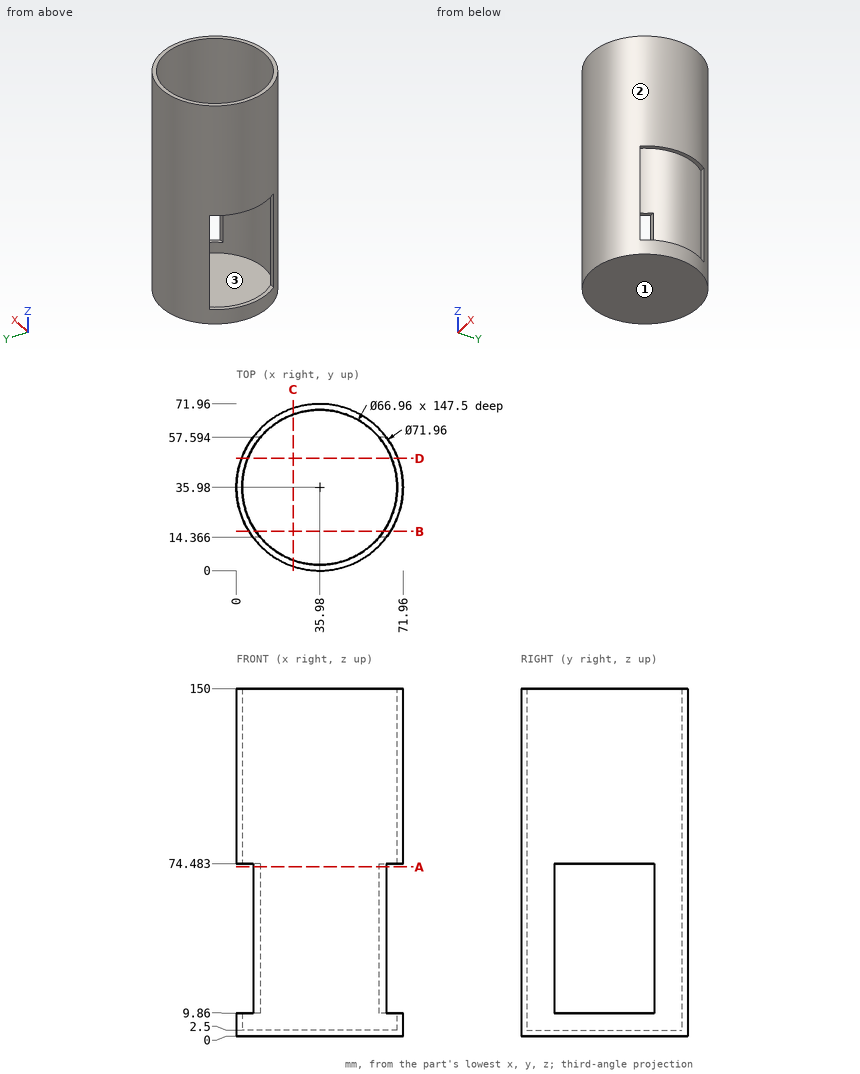
Could you check a few things on this drawing? It's one solid part, dimensions in mm from its lowest x, y, z. Give positions to 0.01 mm unless a question says otherwise; leave off trailing zeros. Order: outer loops, then holes, each group sorted by start corner. A loop starts at its lowest first (then second) coordinate and runs counter-clockwise, first axis right, second up. Notation, with made-up numbers: (-27, 20.5) - (20, 20.5) arc R6 ccw to (20, 29.5) - close; hole circle Ø1 at (64.5, 62). An arc over 180 degrees is marked (long way). Return JSON: item names as keys, results as strings. Group by question number.
Q1. Thinking about a two-plate mould opening in X: for the marked faces 1, 2 and 3, which applies, pulls with the +X half, pulls with the -X half, needs draft (parallel to the pull), parting line crosses it, or undercut?
Q2. Suppose I cut it at A-A, the plane z = 73. Please give me the cut outline in (x, y) (1 decimal).
Q3. Suppose I cut it at B-B, the plane y = 17. Please give me the cut outline in (x, z).
Q4. Suppose I cut it at D-D, the plane y = 48.5. Please give me the cut outline in (x, z).
Q5. Will these pins go through, and if not, where does the flat tip stop? pin 1 Ø2 at (y, z) = (60, 129.5) entering from +X; pin 2 Ø3.5 at (x, z) = (63, 27) entering from -Y; pin 3 Ø2.5 at (x, z) = (9, 35) entering from +Y.
Q6. Please list where these lines run through material, in increasing order: line 1 along Z through (x, y) = (8.5, 14.5); line 2 along Z through (x, y) = (10, 29); line 3 along Y through (x, z) = (25, 38) (1 decimal). Write a range as [from, to].
Q7. Suppose I cut it at C-C, the plane x = 24.5. Please give me the cut outline in (y, z).
Resolved:
{
 "1": {"face 1": "needs draft", "face 2": "parting line crosses it", "face 3": "undercut"},
 "2": {"outline": "(7.2, 14.4) arc R36 ccw to (64.7, 14.4) - (61.5, 14.4) arc R33.5 cw to (10.4, 14.4) - close; (7.2, 57.6) - (10.4, 57.6) arc R33.5 cw to (61.5, 57.6) - (64.7, 57.6) arc R36 ccw to start"},
 "3": {"outline": "(5.41, 0) - (66.55, 0) - (66.55, 9.86) - (63.56, 9.86) - (63.56, 2.5) - (8.4, 2.5) - (8.4, 9.86) - (5.41, 9.86) - close; (5.41, 74.48) - (8.4, 74.48) - (8.4, 150) - (5.41, 150) - close; (63.56, 74.48) - (66.55, 74.48) - (66.55, 150) - (63.56, 150) - close"},
 "4": {"outline": "(2.25, 0) - (69.71, 0) - (69.71, 9.86) - (67.03, 9.86) - (67.03, 2.5) - (4.93, 2.5) - (4.93, 9.86) - (2.25, 9.86) - close; (2.25, 74.48) - (4.93, 74.48) - (4.93, 150) - (2.25, 150) - close; (67.03, 74.48) - (69.71, 74.48) - (69.71, 150) - (67.03, 150) - close"},
 "5": {"pin 1": "stops at x = 63.63", "pin 2": "stops at y = 10.37", "pin 3": "stops at y = 61.13"},
 "6": {"line 1": "z = [0, 9.86], [74.48, 150]", "line 2": "z = [0, 2.5]", "line 3": "y = [1.7, 4.4], [67.6, 70.2]"},
 "7": {"outline": "(1.88, 0) - (70.08, 0) - (70.08, 150) - (67.43, 150) - (67.43, 2.5) - (4.53, 2.5) - (4.53, 150) - (1.88, 150) - close"}
}
